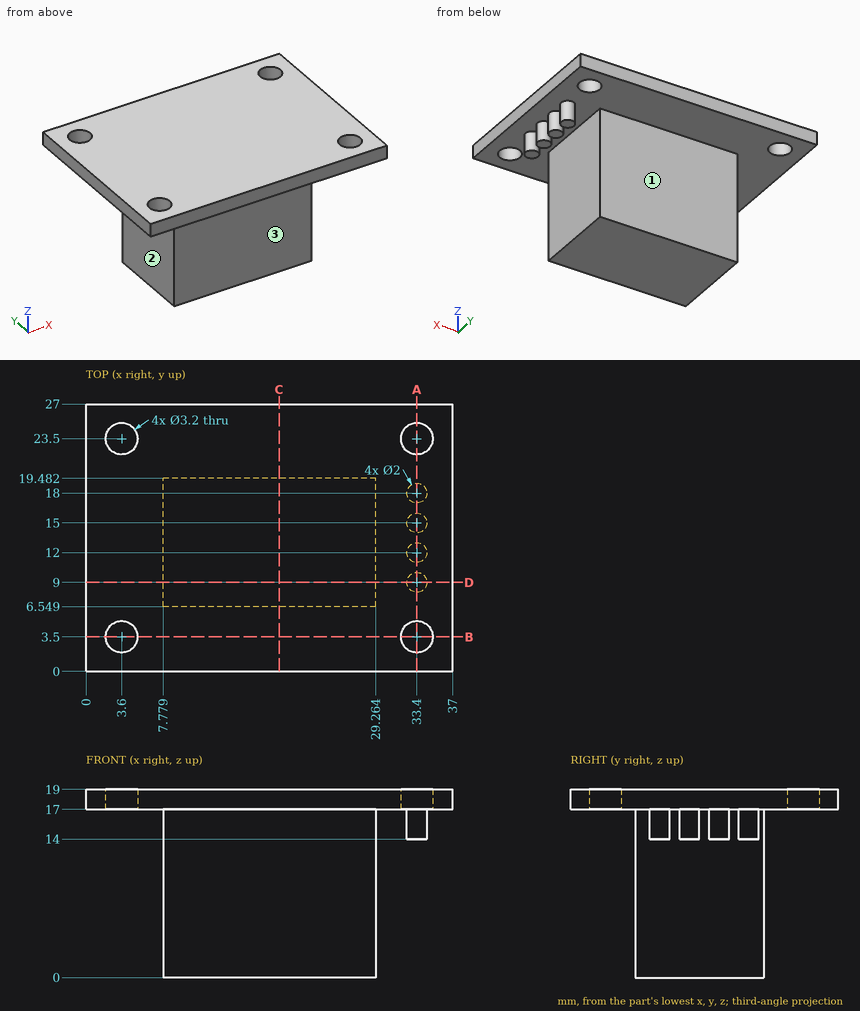
Check sheet for the drawn part. Datum: minimum x, y, z corner. Units: mm. A direction names the side the tool comes from. Give positions to 0.01 mm unless a question says otherwise; leave off trailing zeros. Write each loop counter-clockwise with the first axis right and the second up, starting at its lowest first coordinate (ties: lowest second). Pieces come first, ordered by that corner, then holes.
(1) Cross-section at A-A (x = 33.4). Enter the section's corners in (y, z).
(2) Gauge pin test, flat ends, axial feed: pin 1 (1 mm diameter, centred on y = 6.5, z = 3, fed in from +X); pin 2 (3.5 mm diameter, centred on x = 3.6, y = 3.5, fed in from -Z); pin 3 (4 mm diameter, centred on x = 11, z = 6, fed in from +Y); pin 4 (3.5 mm diameter, centred on x = 33.4, y = 23.5, fed in from +Z). Record the tip position at first contact, or that the pin passes through.
(3) Cross-section at B-B (y = 3.5). Enter the section's corners in (x, z).
(4) Cross-section at C-C (x = 19.5). Enter the section's corners in (y, z), plus the area to 3 significant figures.
(5) Material ranges on line 1 (Y direction, x = 3.6, z = 18.25); line 2 (X direction, y = 14.75, z = 12.5); line 3 (Z direction, x = 27.5, y = 22.5), recorded low to high.
(6) Access from +Z, -Z, +X, -X, +Y, -Y to the whole of each face (thin tool, end or side, straight path). Record for the marked faces 1, 2 and 3.
(7) Cross-section at D-D (y = 9). Enter the section's corners in (x, z).
Worked out:
1. outline: (0, 17) - (1.9, 17) - (1.9, 19) - (0, 19) - close; (5.1, 17) - (8, 17) - (8, 14) - (10, 14) - (10, 17) - (11, 17) - (11, 14) - (13, 14) - (13, 17) - (14, 17) - (14, 14) - (16, 14) - (16, 17) - (17, 17) - (17, 14) - (19, 14) - (19, 17) - (21.9, 17) - (21.9, 19) - (5.1, 19) - close; (25.1, 17) - (27, 17) - (27, 19) - (25.1, 19) - close
2. pin 1: stops at x = 29.26
2. pin 2: stops at z = 17
2. pin 3: stops at y = 19.48
2. pin 4: stops at z = 19
3. outline: (0, 17) - (2, 17) - (2, 19) - (0, 19) - close; (5.2, 17) - (31.8, 17) - (31.8, 19) - (5.2, 19) - close; (35, 17) - (37, 17) - (37, 19) - (35, 19) - close
4. outline: (0, 17) - (6.55, 17) - (6.55, 0) - (19.48, 0) - (19.48, 17) - (27, 17) - (27, 19) - (0, 19) - close
4. area: 274 mm2
5. line 1: y = 0 to 1.9, 5.1 to 21.9, 25.1 to 27
5. line 2: x = 7.78 to 29.26
5. line 3: z = 17 to 19
6. face 1: -Z, +X, -X, +Y
6. face 2: -Z, -X, +Y, -Y
6. face 3: -Z, +X, -X, -Y
7. outline: (0, 17) - (7.78, 17) - (7.78, 0) - (29.26, 0) - (29.26, 17) - (32.4, 17) - (32.4, 14) - (34.4, 14) - (34.4, 17) - (37, 17) - (37, 19) - (0, 19) - close
